from build123d import *

# Parameters (mm, degrees)
SKETCH1_W           = 50
SKETCH1_H           = 130
SKETCH1_R           = 4.108488497
SKETCH1_W_2         = 14
SKETCH1_H_2         = 47.88
BOSS_EXTRUDE1_DEPTH = 1.5
SKETCH2_W           = 1.5
SKETCH2_H           = 130
BOSS_EXTRUDE2_DEPTH = 5
SKETCH3_R           = 1.78890387
CUT_EXTRUDE1_DEPTH  = 83.263296798
FILLET1_R           = 5
FILLET2_R           = 2
SKETCH4_W           = 14
SKETCH4_H           = 1.5
BOSS_EXTRUDE3_DEPTH = 20
FILLET3_R           = 6
FILLET4_R           = 1
SKETCH5_R           = 5
CUT_EXTRUDE2_DEPTH  = 97.263407498


with BuildPart() as part:
    # Sketch1 → Boss-Extrude1 (new body)
    with BuildSketch(Plane.XY):
        Rectangle(SKETCH1_W, SKETCH1_H)
        with Locations((0, 43.4034135)):
            Circle(SKETCH1_R, mode=Mode.SUBTRACT)
        with Locations(Location((0, -43.4034135, 0), (0, 0, 180))):
            Circle(SKETCH1_R, mode=Mode.SUBTRACT)
        Rectangle(SKETCH1_W_2, SKETCH1_H_2, mode=Mode.SUBTRACT)
        with BuildLine():
            Line((9.165030278, 51.424748184), (-9.165030278, 51.424748184))
            ThreePointArc((-9.165030278, 51.424748184), (-13.077876466, 55.337594372), (-9.165030278, 59.250440559))
            Line((-9.165030278, 59.250440559), (9.165030278, 59.250440559))
            ThreePointArc((9.165030278, 59.250440559), (13.077876466, 55.337594372), (9.165030278, 51.424748184))
        make_face(mode=Mode.SUBTRACT)
        with BuildLine():
            Line((9.165030278, -51.424748184), (-9.165030278, -51.424748184))
            ThreePointArc((-9.165030278, -51.424748184), (-13.077876466, -55.337594372), (-9.165030278, -59.250440559))
            Line((-9.165030278, -59.250440559), (9.165030278, -59.250440559))
            ThreePointArc((9.165030278, -59.250440559), (13.077876466, -55.337594372), (9.165030278, -51.424748184))
        make_face(mode=Mode.SUBTRACT)
    extrude(amount=BOSS_EXTRUDE1_DEPTH)

    # Sketch2 → Boss-Extrude2 (add)
    with BuildSketch(Plane.XY.offset(1.5)):
        with Locations((-24.25, 0)):
            Rectangle(SKETCH2_W, SKETCH2_H)
        with Locations((24.25, 0)):
            Rectangle(SKETCH2_W, SKETCH2_H)
    extrude(amount=BOSS_EXTRUDE2_DEPTH)

    # Sketch3 → Cut-Extrude1 (cut, through all)
    with BuildSketch(Plane(origin=(25, 0, 0), x_dir=(0, 0, -1), z_dir=(1, 0, 0))):
        with Locations((-3.509314499, 51.836194759)):
            Circle(SKETCH3_R)
        with Locations(Location((-3.509314499, -51.836194759, 0), (0, 0, 90))):
            Circle(SKETCH3_R)
    extrude(amount=-CUT_EXTRUDE1_DEPTH, mode=Mode.SUBTRACT)

    # Fillet1
    fillet1_edges = [part.edges().sort_by_distance(p)[0] for p in [
        (-24.25, -65, 6.5),
        (24.25, -65, 6.5),
        (24.25, 65, 6.5),
        (-24.25, 65, 6.5),
    ]]
    fillet(fillet1_edges, radius=FILLET1_R)

    # Fillet2
    # the kernel refuses this fillet: 2 mm, written as the material it takes off along each edge
    with BuildSketch(Plane(origin=(25, 70, 0), x_dir=(0, 0, 1), z_dir=(0, -1, 0))) as fillet2_piece_1:
        with BuildLine():
            CenterArc((FILLET2_R, FILLET2_R), FILLET2_R, 180, 90)
            Line((0, FILLET2_R), (0, 0))
            Line((0, 0), (FILLET2_R, 0))
        make_face()
    extrude(amount=140, mode=Mode.SUBTRACT)
    with BuildSketch(Plane(origin=(-25, -70, 0), x_dir=(1, 0, 0), z_dir=(0, 1, 0))) as fillet2_piece_2:
        with BuildLine():
            CenterArc((FILLET2_R, -FILLET2_R), FILLET2_R, 90, 90)
            Line((0, -FILLET2_R), (0, 0))
            Line((0, 0), (FILLET2_R, 0))
        make_face()
    extrude(amount=140, mode=Mode.SUBTRACT)

    # Sketch4 → Boss-Extrude3 (add)
    with BuildSketch(Plane.XY.offset(1.5)):
        with Locations((0, 24.69)):
            Rectangle(SKETCH4_W, SKETCH4_H)
        with Locations((0, -24.69)):
            Rectangle(SKETCH4_W, SKETCH4_H)
    extrude(amount=BOSS_EXTRUDE3_DEPTH)

    # Fillet3
    fillet3_edges = [part.edges().sort_by_distance(p)[0] for p in [
        (7, 24.69, 21.5),
        (-7, 24.69, 21.5),
        (-7, -24.69, 21.5),
        (7, -24.69, 21.5),
    ]]
    fillet(fillet3_edges, radius=FILLET3_R)

    # Fillet4
    fillet4_edges = [part.edges().sort_by_distance(p)[0] for p in [
        (0, -23.94, 0),
        (0, 23.94, 0),
        (0, 25.44, 1.5),
        (0, -25.44, 1.5),
    ]]
    fillet(fillet4_edges, radius=FILLET4_R)

    # Sketch5 → Cut-Extrude2 (cut, through all)
    with BuildSketch(Plane(origin=(0, 25.44, 0), x_dir=(1, 0, 0), z_dir=(0, 1, 0))):
        with Locations(Location((0, -13.904712179, 0), (0, 0, 180))):
            Circle(SKETCH5_R)
    extrude(amount=-CUT_EXTRUDE2_DEPTH, mode=Mode.SUBTRACT)


solid = part.part
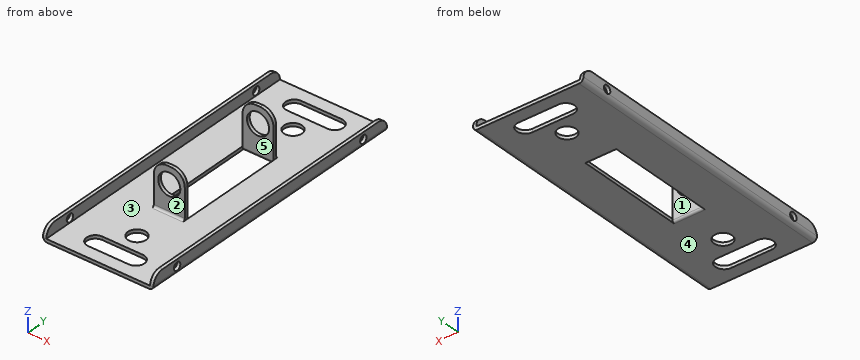
For this review, take the finished solid that the model builds, in its own axes (mm). Face numbers are marked on the shaded views. A direction names the side the tool comes from. Round coordinates to 2 decimals unless told otherwise and drop trailing zeros. Write each loop counter-clockwise with the first axis right and the second up, starting at its lowest first coordinate (ties: lowest second). Pieces come first, ordered by that corner, then holes. Notation, with made-up numbers: (4, 82) - (43, 82) arc R34 ccw to (43, 121) - close; hole circle Ø10 at (53, -14.75). An arc over 180 degrees is marked (long way). Use a Markdown table: item, result.
Q1. The part is to be moulded in two halves that separate along X. For the marked faces 3, 4 and 5, say which applies: pulls with the +X half, pulls with the -X half, needs draft (parallel to the pull), parting line crosses it, or undercut.
Derived:
| item | result |
|---|---|
| face 3 | undercut |
| face 4 | needs draft |
| face 5 | undercut |
Q2. Clearance check with flat-ended pins moving along their axes: pin 1 (6 mm diameter, centred on x = 0, z = 13.9, fed in from -Y); pin 2 (10.5 mm diameter, centred on x = 0, y = 43.4, fed in from -Z); pin 3 (6 mm diameter, centred on x = -2, z = 17, fed in from +Y); pin 4 (10 mm diameter, centred on x = -11, y = -26.5, fed in from +Z). State where each tip first meets the part, or that it passes through.
Derived:
| item | result |
|---|---|
| pin 1 | passes through |
| pin 2 | stops at z = 0 |
| pin 3 | stops at y = 25.44 |
| pin 4 | stops at z = 18.64 |
Q3. Machinability: for the marked faces 1 and 2, which of the approach directions +Z, -Z, +X, -X, +Y, -Y give a long, thin tool a straight path to every point of the face, cutting with its end or side? Answer none if there is none.
Derived:
| item | result |
|---|---|
| face 1 | +Z, -Z |
| face 2 | +Z, -Y |
Q4. Wall thickness on line 1 along Y through (x, z) = (0, 1); line 2 along Y through (x, z) = (-6.5, 10); line 3 along X through (y, z) = (23, 5.5): over which ranges is each line inside the solid? List them lowest first.
Derived:
| item | result |
|---|---|
| line 1 | y = -65 to -59.25, -51.42 to -47.51, -39.29 to -23.94, 23.94 to 39.29, 47.51 to 51.42, 59.25 to 65 |
| line 2 | y = -25.44 to -23.94, 23.94 to 25.44 |
| line 3 | x = -25 to -23.5, 23.5 to 25 |
Q5. We need section B-B (z = 11). Give the boundary of the cut face in (x, y), plus the area to 3 significant figures.
Derived:
| item | result |
|---|---|
| outline | (-7, -25.44) - (-4.07, -25.44) - (-4.07, -23.94) - (-7, -23.94) - close; (-7, 23.94) - (-4.07, 23.94) - (-4.07, 25.44) - (-7, 25.44) - close; (4.07, -25.44) - (7, -25.44) - (7, -23.94) - (4.07, -23.94) - close; (4.07, 23.94) - (7, 23.94) - (7, 25.44) - (4.07, 25.44) - close |
| area | 17.6 mm2 |
Q6. We need section A-A (y = -13). Give the boundary of the cut face in (x, z).
Derived:
| item | result |
|---|---|
| outline | (-25, 2) arc R2 ccw to (-23, 0) - (-7, 0) - (-7, 1.5) - (-23.5, 1.5) - (-23.5, 6.5) - (-25, 6.5) - close; (7, 0) - (23, 0) arc R2 ccw to (25, 2) - (25, 6.5) - (23.5, 6.5) - (23.5, 1.5) - (7, 1.5) - close |
